Geometry check sheet. Reference: drawing and pictorial views, mm from the part's lowest x, y, z. A direction names the side the tool comes from. Coordinates: 2 decimals unless noted, no trailing zeros. Write each loop counter-clockwise with the first axis right and the second up, starting at its lowest first coordinate (ties: lowest second). Pieces come first, ordered by that corner, then holes.
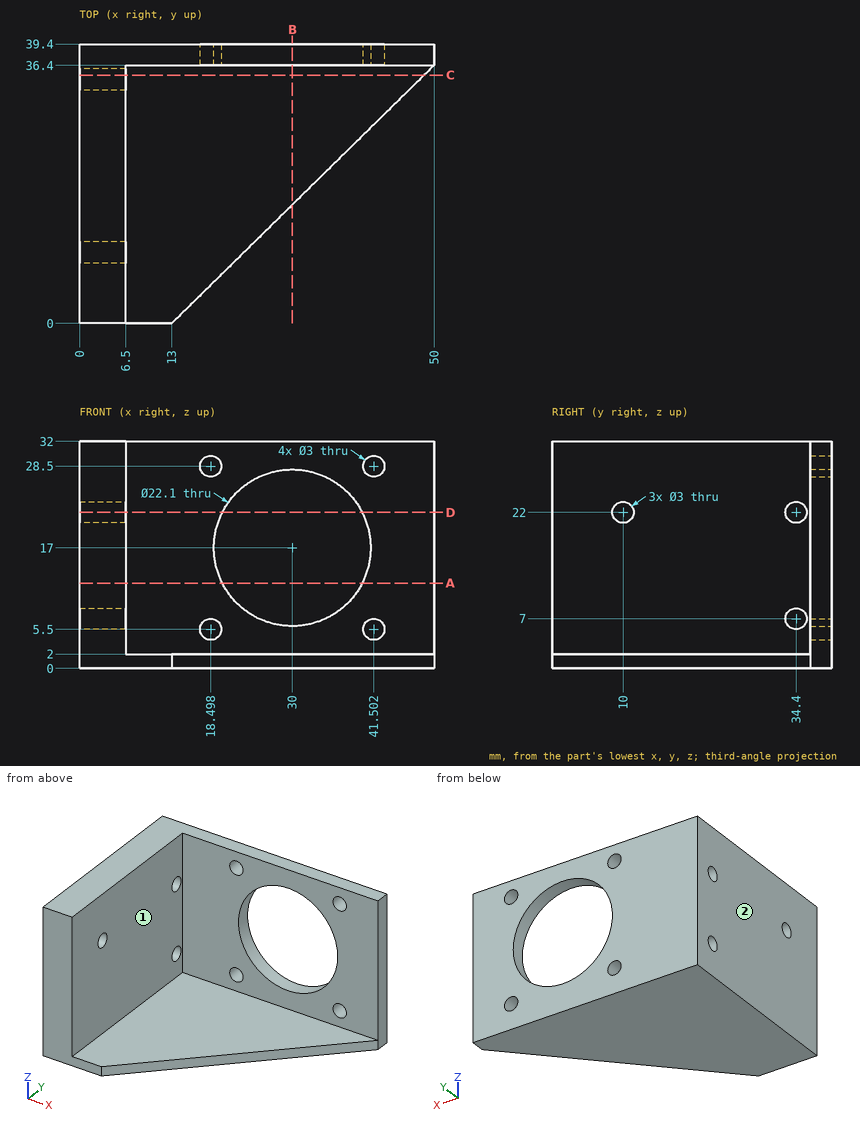
1. Sectioned sample at D-D, the plane z = 22. Record the boundary of the cut face in (x, y).
2. Sectioned sample at C-C, the plane y = 35. Record the boundary of the cut face in (x, z) (1 decimal), and give its area (3 significant figures).
3. Tool access check on the marked faces 1 and 2. Record the directions out of +Z, -Z, +X, -X, +Y, -Y that give a thin tool (end or side, any length) a straight path to the whole face; none if there is none.
4. Sectioned sample at A-A, the plane z = 12. Record the boundary of the cut face in (x, y).
5. Gauge pin test, flat ends, axial feed: P1, Ø1, axis at x = 25.5, y = 9.5, coming from the +Z side; P2, Ø10, axis at x = 39, y = 19, coming from the +Z side; P3, Ø1, axis at y = 9, z = 23, coming from the +X side; P4, Ø5, axis at y = 14, z = 3.5, coming from the +X side. Record the tip position at first contact, or that the pin passes through.
6. Material ranges on L1, parallel to X at y = 38.8, z = 28.5; L2, parallel to Y at x = 1, z = 22; L3, parallel to X at y = 9.5, z = 19.5, recorded low to high.
7. Sectioned sample at B-B, the plane x = 30. Record the boundary of the cut face in (y, z).
Outcome:
1. outline: (0, 0) - (6.5, 0) - (6.5, 8.5) - (0, 8.5) - close; (0, 11.5) - (6.5, 11.5) - (6.5, 32.9) - (0, 32.9) - close; (0, 35.9) - (6.5, 35.9) - (6.5, 36.4) - (20.15, 36.4) - (20.15, 39.4) - (0, 39.4) - close; (39.85, 36.4) - (50, 36.4) - (50, 39.4) - (39.85, 39.4) - close
2. outline: (0, 0) - (48.6, 0) - (48.6, 2) - (6.5, 2) - (6.5, 5.6) - (0, 5.6) - close; (0, 8.4) - (6.5, 8.4) - (6.5, 20.6) - (0, 20.6) - close; (0, 23.4) - (6.5, 23.4) - (6.5, 32) - (0, 32) - close
2. area: 256 mm2
3. face 1: +Z, +X, -Y
3. face 2: +Z, -Z, -X, +Y, -Y
4. outline: (0, 0) - (6.5, 0) - (6.5, 36.4) - (20.15, 36.4) - (20.15, 39.4) - (0, 39.4) - close; (39.85, 36.4) - (50, 36.4) - (50, 39.4) - (39.85, 39.4) - close
5. P1: passes through
5. P2: stops at z = 2
5. P3: stops at x = 6.5
5. P4: stops at x = 29.26
6. L1: x = 0 to 17, 20 to 40, 43 to 50
6. L2: y = 0 to 8.5, 11.5 to 32.9, 35.9 to 39.4
6. L3: x = 0 to 6.5
7. outline: (16.72, 0) - (39.4, 0) - (39.4, 5.95) - (36.4, 5.95) - (36.4, 2) - (16.72, 2) - close; (36.4, 28.05) - (39.4, 28.05) - (39.4, 32) - (36.4, 32) - close
